from build123d import *

# Parameters (mm, degrees)
SKETCH_1_R      = 10
EXTRUDE_1_DEPTH = 20
EXTRUDE_2_DEPTH = 35


with BuildPart() as part:
    # Эскиз1 → Бобышка-Вытянуть1 (new body)
    with BuildSketch(Plane.XY):
        with BuildLine():
            Line((-50, -25.617376915), (-50, -35))
            Line((-50, -35), (50, -35))
            Line((50, -35), (50, 35))
            Line((50, 35), (-50, 35))
            Line((-50, 35), (-50, 25.617376915))
            ThreePointArc((-50, 25.617376915), (-67.5, 0), (-50, -25.617376915))
        make_face()
        with Locations((-40, 0)):
            Circle(SKETCH_1_R, mode=Mode.SUBTRACT)
    extrude(amount=EXTRUDE_1_DEPTH)

    # Эскиз2 → Бобышка-Вытянуть2 (add)
    with BuildSketch(Plane.ZY.offset(20)):
        Polygon((0, 35), (0, -35), (40, -35), (40, -22.5), (30, -22.5), (30, -12.5), (25, -12.5), (25, 12.5), (30, 12.5), (30, 22.5), (40, 22.5), (40, 35), align=None)
    extrude(amount=-EXTRUDE_2_DEPTH)


solid = part.part
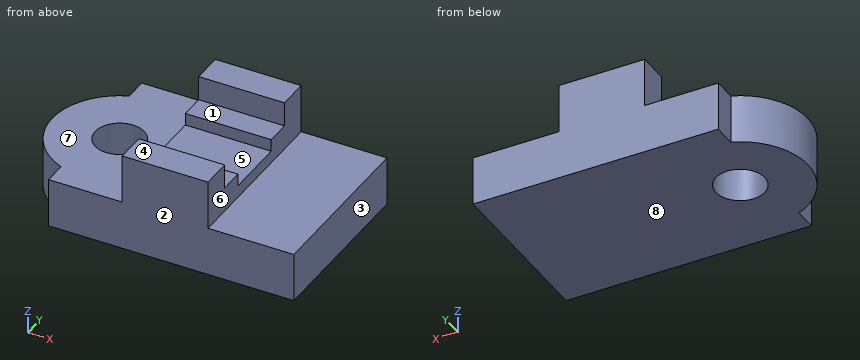
Verification items for the finished model (mm, model axes). Face numbers are marked on the shaded views. A direction names the side the tool comes from. Give positions to 0.01 mm unless a question says otherwise; leave off trailing zeros. Loops run counter-clockwise (first coordinate to the right, second up) from the corner with the lowest first, then second, coordinate; pieces in that order, holes last.
1) Sectioned sample at B-B, the plane x = -40. Enter the section's corners in (y, z).
2) Set-up check for the marked faces 4, 5, 6, 7 and 8: record each of +Z, -Z, +X, -X, +Y, -Y from which the full face is reachable in a straight line by a thin tool's end or side.
3) Draft check along Y on the marked faces 1, 2 and 3. Enter one of: pulls with the +Y half, pulls with the -Y half, needs draft (parallel to the pull), parting line crosses it, or undercut.
4) Sectioned sample at C-C, the plane z = 27.5. Enter the section's corners in (x, y), then the cut area to 4 significant figures.
5) Sectioned sample at D-D, the plane x = 13. Enter the section's corners in (y, z).
6) Thickness scan on line 1 along Y through (x, z) = (-40, 5); line 2 along Z through (x, y) = (-55.5, 20); line 3 along X through (y, z) = (26.5, 30). Record the ranges inside material, lowest first.
7) Sectioned sample at A-A, the plane y = 0. Enter the section's corners in (x, z).
8) Depth check by flat-ended pin: pin 1 Ø8 at (x, y) = (-20.5, -25) entering from -Z; pin 2 Ø16 at (y, z) = (-17, 30.5) entering from +X; pin 3 Ø16 at (x, y) = (-40, 0) entering from +Z; pin 4 Ø8 at (y, z) = (11, 25.5) entering from -X. Enter the tip coordinate at first touch or a pass-through.
Answers:
1. outline: (-35, 0) - (-10, 0) - (-10, 20) - (-35, 20) - close; (10, 0) - (35, 0) - (35, 20) - (10, 20) - close
2. face 4: +Z, +X, -X, +Y, -Y
2. face 5: +Z, +X, -X
2. face 6: +Z, +X, +Y, -Y
2. face 7: +Z, -X, +Y, -Y
2. face 8: -Z, +X, -X, +Y, -Y
3. face 1: undercut
3. face 2: pulls with the -Y half
3. face 3: needs draft
4. outline: (-20, -35) - (15, -35) - (15, -12.5) - (-20, -12.5) - close; (-20, 12.5) - (15, 12.5) - (15, 35) - (-20, 35) - close
4. area: 1,575 mm2
5. outline: (-35, 0) - (35, 0) - (35, 40) - (22.5, 40) - (22.5, 30) - (12.5, 30) - (12.5, 25) - (-12.5, 25) - (-12.5, 30) - (-22.5, 30) - (-22.5, 40) - (-35, 40) - close
6. line 1: y = -35 to -10, 10 to 35
6. line 2: z = 0 to 20
6. line 3: x = -20 to 15
7. outline: (-67.5, 0) - (-50, 0) - (-50, 20) - (-67.5, 20) - close; (-30, 0) - (50, 0) - (50, 20) - (15, 20) - (15, 25) - (-20, 25) - (-20, 20) - (-30, 20) - close
8. pin 1: stops at z = 0
8. pin 2: stops at x = 15
8. pin 3: passes through
8. pin 4: stops at x = -20
